Verification items for this drawing (mm, ordinates from the low corner). A direction names the side the tool comes from. Give positions to 0.01 mm unless a question says otherwise; leave off trailing zeros. Order: outer loops, then holes, each group sorted by start corner. A loop starts at its lowest first (then second) coordinate and runs counter-clockwise, first axis right, second up.
(1) Sectioned sample at C-C on y = 1.75. Record the cut outline in (x, z), plus the area to 3 significant figures.
(2) Access from +Z, -Z, +X, -X, +Y, -Y to the whole of each face (thin tool, end or side, straight path). Record for the marked faces 3 and 4.
(3) Sectioned sample at D-D on x = 48. Record the cut outline in (y, z), plus the area to 3 significant figures.
(4) Sectioned sample at B-B on x = 26. Record the cut outline in (y, z).
(5) Mould release check, pull along Z, two halves, no side actions. Record for the marked faces 1 and 2: pulls with the +Z half, pulls with the -Z half, needs draft (parallel to the pull), parting line crosses it, or undercut.
(6) Scan lines: L1, parallel to X at y = 14.55, z = 26; L2, parallel to X at y = 14.75, z = 22; L3, parallel to X at y = 6.25, z = 26. Record each from-to range of solid material in increasing order.
(7) Gauge pin test, flat ends, axial feed: pin 1 (1 mm diameter, centred on y = 8, z = 18, fed in from +X); pin 2 (4 mm diameter, centred on y = 9, z = 42.5, fed in from -X); pin 3 (8 mm diameter, centred on x = 44.5, y = 10.5, fed in from +Z). Record the tip position at first contact, or that the pin passes through.
(8) Sectioned sample at A-A on z = 26. Record the cut outline in (x, y).
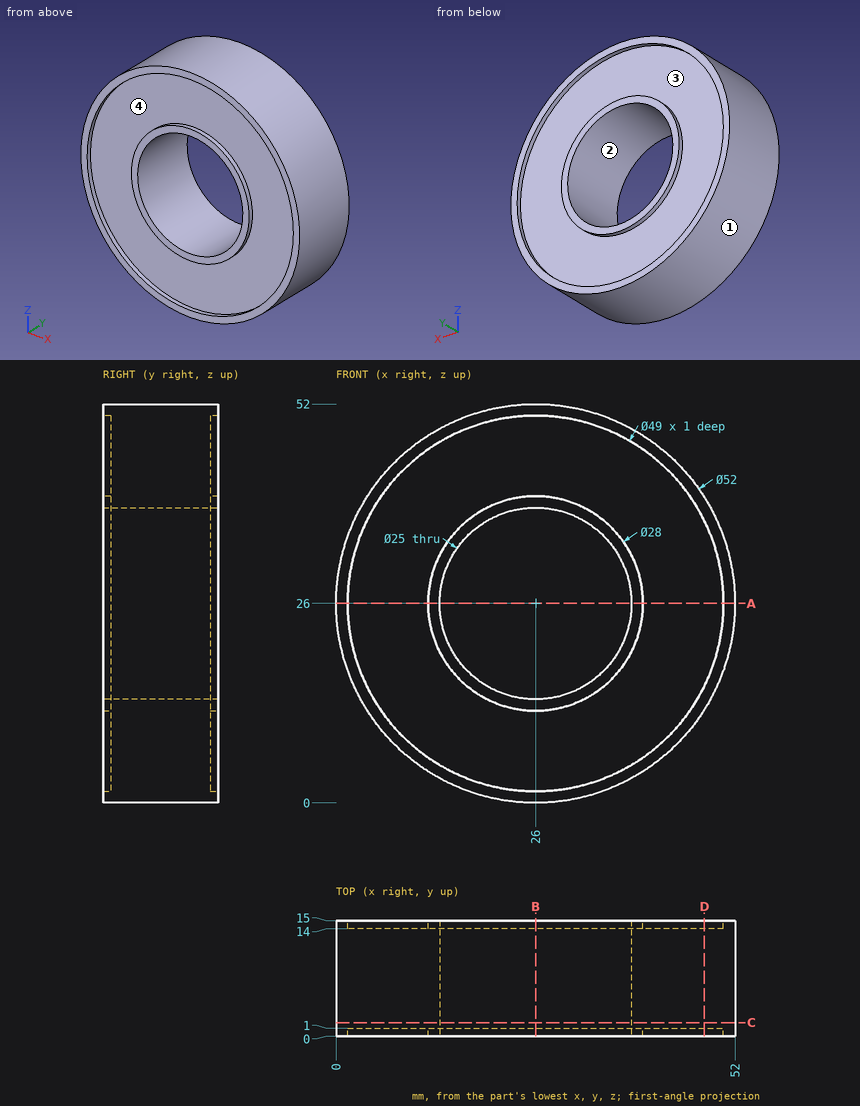
Ans:
1. outline: circle Ø52 at (26, 26); hole circle Ø25 at (26, 26)
1. area: 1,630 mm2
2. face 3: +Y
2. face 4: -Y
3. outline: (0, 12.14) - (15, 12.14) - (15, 15.22) - (14, 15.22) - (14, 36.78) - (15, 36.78) - (15, 39.86) - (0, 39.86) - (0, 36.78) - (1, 36.78) - (1, 15.22) - (0, 15.22) - close
3. area: 373 mm2
4. outline: (0, 0) - (15, 0) - (15, 1.5) - (14, 1.5) - (14, 12) - (15, 12) - (15, 13.5) - (0, 13.5) - (0, 12) - (1, 12) - (1, 1.5) - (0, 1.5) - close; (0, 38.5) - (15, 38.5) - (15, 40) - (14, 40) - (14, 50.5) - (15, 50.5) - (15, 52) - (0, 52) - (0, 50.5) - (1, 50.5) - (1, 40) - (0, 40) - close
5. face 1: parting line crosses it
5. face 2: undercut
6. L1: x = 0 to 1.5, 12 to 13.5, 38.5 to 40, 50.5 to 52
6. L2: x = 0.31 to 1.83, 12.58 to 14.16, 37.84 to 39.42, 50.17 to 51.69
6. L3: x = 0 to 13.5, 38.5 to 52
7. pin 1: stops at x = 50.89
7. pin 2: stops at x = 4.42
7. pin 3: stops at z = 47.58
8. outline: (0, 0) - (1.5, 0) - (1.5, 1) - (12, 1) - (12, 0) - (13.5, 0) - (13.5, 15) - (12, 15) - (12, 14) - (1.5, 14) - (1.5, 15) - (0, 15) - close; (38.5, 0) - (40, 0) - (40, 1) - (50.5, 1) - (50.5, 0) - (52, 0) - (52, 15) - (50.5, 15) - (50.5, 14) - (40, 14) - (40, 15) - (38.5, 15) - close
